Geometry check sheet. Reference: the model listing, model coordinates, mm. Face numbers are marked on the shaded views. A direction names the side the tool comes from. Give positions to 0.01 mm unless a question says otherwise; leave off trailing zeros. Write each loop counter-clockwise with the first axis right and the second up, starting at its lowest first coordinate (ties: lowest second). Pieces come first, ordered by that corner, then holes. Notation, with made-up numbers: (42, 28) - (69, 28) arc R12 ccw to (69, 45) - close; hole circle Ø11 at (68.25, 64.25). An arc over 180 degrees is marked (long way). Write item = value, one per line. Start each with the question number.
(1) Thickness scan on L1, parallel to Y at x = 7, z = 38.5; L2, parallel to X at y = 0, z = 8.5; L3, parallel to X at y = -11.25, z = 38. Record the ranges inside material, lowest first.
(2) Access from +Z, -Z, +X, -X, +Y, -Y to the whole of each face (thin tool, end or side, straight path). Record for the marked faces 1 and 2.
(3) Depth check by flat-ended pin: pin 1 Ø9 at (x, z) = (0, 38) entering from +Y; pin 2 Ø2 at (x, z) = (4.5, 6) entering from +Y; pin 3 Ø1.5 at (x, z) = (-5, 12.5) entering from +Y. Enter the tip coordinate at first touch or a pass-through.
(4) Section check B-B, the plane x = 0. Enter the section's corners in (y, z), plus the area to 3 significant figures.
(5) Section check A-A, the plane z = 23. Enter the section's corners in (x, y), plus the area to 3 significant figures.
(6) Draft check along X on the marked faces 3, 4, 5 and 6. Enter one of: pulls with the +X half, pulls with the -X half, needs draft (parallel to the pull), parting line crosses it, or undercut.
(7) Section check C-C, the plane y = 0. Enter the section's corners in (x, z).
(8) Section check D-D, the plane x = 4. Enter the section's corners in (y, z).
```python
from build123d import *

# Parameters (mm, degrees)
SKETCH1_W                = 22
SKETCH1_H                = 27
EXTRUDE1_DEPTH           = 60
EXTRUDE2_DEPTH           = 12
EXTRUDE2_DEPTH_BACK      = 12
SKETCH3_R                = 5
EXTRUDE3_DEPTH           = 14.5
EXTRUDE3_DEPTH_BACK      = 14.5
F_5_16_24_TAPPED_HOLE2_D = 6.9088
CUT_EXTRUDE1_DEPTH       = 9.0000001
CUT_EXTRUDE1_DEPTH_BACK  = 9.0000001
FILLET2_R                = 3


with BuildPart() as part:
    # Sketch1 → Extrude1 (new body)
    with BuildSketch(Plane.XY):
        Rectangle(SKETCH1_W, SKETCH1_H)
    extrude(amount=EXTRUDE1_DEPTH)

    # Sketch2 → Extrude2 (cut, two sides)
    with BuildSketch(Plane(origin=(0, 0, 0), x_dir=(0, 0, -1), z_dir=(1, 0, 0))) as extrude2_sk:
        with BuildLine():
            Line((-66.910918786, 10), (-21, 10))
            ThreePointArc((-21, 10), (-11, 0), (-21, -10))
            Line((-21, -10), (-66.910918786, -10))
            Line((-66.910918786, -10), (-66.910918786, 10))
        make_face()
    extrude(amount=EXTRUDE2_DEPTH, mode=Mode.SUBTRACT)
    extrude(extrude2_sk.sketch, amount=-EXTRUDE2_DEPTH_BACK, mode=Mode.SUBTRACT)

    # Sketch3 → Extrude3 (cut, two sides)
    with BuildSketch(Plane(origin=(0, 0, 0), x_dir=(1, 0, 0), z_dir=(0, 1, 0))) as extrude3_sk:
        with Locations((0, -38)):
            Circle(SKETCH3_R)
        with BuildLine():
            Line((-8, -38), (-8, 11.717299326))
            Line((-8, 11.717299326), (-29.903870298, 11.717299326))
            Line((-29.903870298, 11.717299326), (-29.903870298, -74.658770221))
            Line((-29.903870298, -74.658770221), (37.768949852, -74.658770221))
            Line((37.768949852, -74.658770221), (37.768949852, 11.717299326))
            Line((37.768949852, 11.717299326), (8, 11.717299326))
            Line((8, 11.717299326), (8, -38))
            ThreePointArc((8, -38), (0, -46), (-8, -38))
        make_face()
    extrude(amount=EXTRUDE3_DEPTH, mode=Mode.SUBTRACT)
    extrude(extrude3_sk.sketch, amount=-EXTRUDE3_DEPTH_BACK, mode=Mode.SUBTRACT)

    # 5_16-24 Tapped Hole2 (through all)
    with Locations(Plane(origin=(0, 0, 0), x_dir=(-1, 0, 0), z_dir=(0, 0, -1))):
        with Locations((0, 0)):
            Hole(F_5_16_24_TAPPED_HOLE2_D / 2)

    # Sketch8 → Cut-Extrude1 (cut, two sides)
    with BuildSketch(Plane(origin=(0, 0, 0), x_dir=(0, 0, -1), z_dir=(1, 0, 0))) as cut_extrude1_sk:
        Polygon((0, -6), (0, 6), (-17.643434352, 16.186441572), (9.090258644, 16.186441572), (9.090258644, -16.186441572), (-17.643434352, -16.186441572), align=None)
    extrude(amount=CUT_EXTRUDE1_DEPTH, mode=Mode.SUBTRACT)
    extrude(cut_extrude1_sk.sketch, amount=-CUT_EXTRUDE1_DEPTH_BACK, mode=Mode.SUBTRACT)

    # Fillet2
    fillet2_edges = [part.edges().sort_by_distance(p)[0] for p in [
        (-8, 9.75, 6.495190528),
        (8, 9.75, 6.495190528),
        (8, -9.75, 6.495190528),
        (0, 13.5, 12.990381057),
        (-8, -9.75, 6.495190528),
        (0, -13.5, 12.990381057),
    ]]
    fillet(fillet2_edges, radius=FILLET2_R)


solid = part.part
```
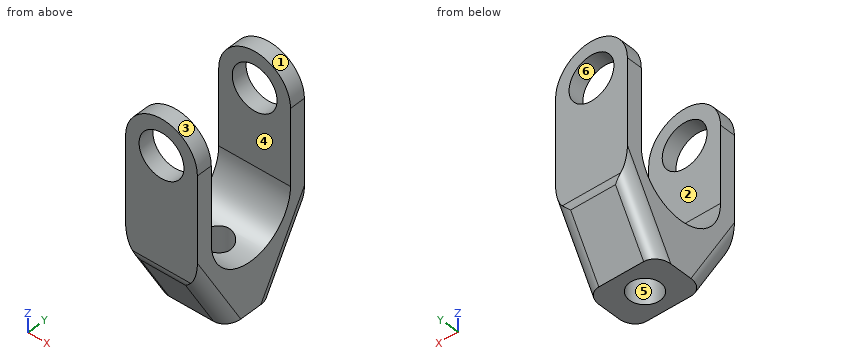
Model answer:
q1.L1 = -13.5 to -10, 10 to 13.5
q1.L2 = -8 to -3.45, 3.45 to 8
q1.L3 = -8 to -5, 5 to 8
q2.face_1 = +Z, +Y, -Y
q2.face_2 = +Z, +X, -X
q3.pin_1 = through
q3.pin_2 = 10.04
q3.pin_3 = 13.45
q4.outline = (-13.5, 13.79) arc R3 ccw to (-13.1, 12.29) - (-6, 0) - (-3.45, 0) - (-3.45, 11.62) arc R10 cw to (-10, 21) - (-10, 33) - (-13.5, 33) - close; (-13.5, 43) - (-10, 43) - (-10, 46) - (-13.5, 46) - close; (3.45, 0) - (6, 0) - (13.1, 12.29) arc R3 ccw to (13.5, 13.79) - (13.5, 33) - (10, 33) - (10, 21) arc R10 cw to (3.45, 11.62) - close; (10, 43) - (13.5, 43) - (13.5, 46) - (10, 46) - close
q4.area = 340 mm²
q5.outline = (-8, -13.5) - (8, -13.5) - (8, -10) - (-8, -10) - close; (-8, 10) - (8, 10) - (8, 13.5) - (-8, 13.5) - close
q5.area = 112 mm²
q6.face_3 = parting line crosses it
q6.face_4 = needs draft
q6.face_5 = undercut
q6.face_6 = undercut
q7.outline = (-8, 0) - (-3.45, 0) - (-3.45, 11) - (-8, 11) - close; (3.45, 0) - (8, 0) - (8, 11) - (3.45, 11) - close
q8.outline = (-13.5, 13.79) arc R3 ccw to (-13.1, 12.29) - (-6, 0) - (6, 0) - (13.1, 12.29) arc R3 ccw to (13.5, 13.79) - (13.5, 35) - (10, 35) - (10, 21) arc R10 cw to (-10, 21) - (-10, 35) - (-13.5, 35) - close; (-13.5, 41) - (-10, 41) - (-10, 44.93) - (-13.5, 44.93) - close; (10, 41) - (13.5, 41) - (13.5, 44.93) - (10, 44.93) - close
